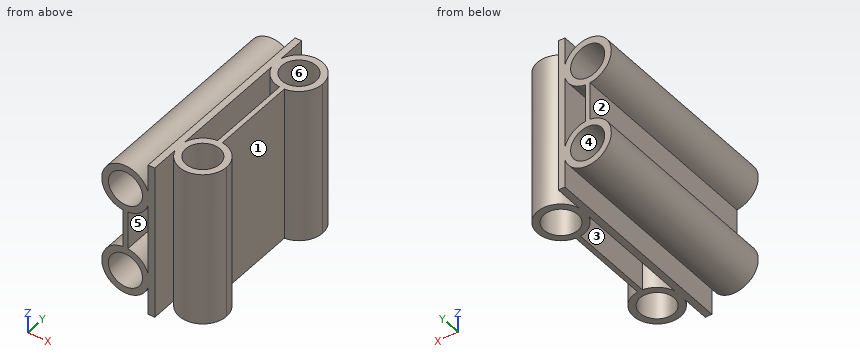
```python
from build123d import *

# Parameters (mm, degrees)
F2_W          = 7
F2_H          = 214
F3_DEPTH      = 82
F3_DEPTH_BACK = 82
F0_R          = 18
F4_DEPTH      = 107
F4_DEPTH_BACK = 107
F1_R          = 18
F5_DEPTH      = 82
F5_DEPTH_BACK = 82


with BuildPart() as f3:
    # F2 (on Top) → F3 (new body, two sides)
    with BuildSketch(Plane.XY) as f3_sk:
        with Locations((-27.5, 0)):
            Rectangle(F2_W, F2_H)
    extrude(amount=F3_DEPTH)
    extrude(f3_sk.sketch, amount=-F3_DEPTH_BACK)

    # F0 (on Front) → F4 (join, two sides)
    with BuildSketch(Plane.XZ) as f4_sk:
        with BuildLine():
            ThreePointArc((-52.5, 20.125314), (-36.459504, 28.22949), (-30, 45))
            ThreePointArc((-30, 45), (-71.77051, 63.540496), (-57.5, 20.125314))
            Line((-57.5, 20.125314), (-52.5, 20.125314))
        make_face()
        with Locations((-55, 45)):
            Circle(F0_R, mode=Mode.SUBTRACT)
        with BuildLine():
            Line((-52.5, -20.125314), (-57.5, -20.125314))
            ThreePointArc((-57.5, -20.125314), (-71.77051, -63.540496), (-30, -45))
            ThreePointArc((-30, -45), (-36.459504, -28.22949), (-52.5, -20.125314))
        make_face()
        with Locations((-55, -45)):
            Circle(F0_R, mode=Mode.SUBTRACT)
        with BuildLine():
            Line((-52.5, 20.125314), (-57.5, 20.125314))
            ThreePointArc((-57.5, 20.125314), (-55, 20), (-52.5, 20.125314))
        make_face()
        with BuildLine():
            ThreePointArc((-52.5, 20.125314), (-55, 20), (-57.5, 20.125314))
            Line((-57.5, 20.125314), (-57.5, -20.125314))
            ThreePointArc((-57.5, -20.125314), (-55, -20), (-52.5, -20.125314))
            Line((-52.5, -20.125314), (-52.5, 20.125314))
        make_face()
        with BuildLine():
            ThreePointArc((-52.5, -20.125314), (-55, -20), (-57.5, -20.125314))
            Line((-57.5, -20.125314), (-52.5, -20.125314))
        make_face()
    extrude(amount=F4_DEPTH)
    extrude(f4_sk.sketch, amount=-F4_DEPTH_BACK)

    # F1 (on Top) → F5 (join, two sides)
    with BuildSketch(Plane.XY) as f5_sk:
        with BuildLine():
            ThreePointArc((2.5, 45.125314), (18.540496, 53.22949), (25, 70))
            ThreePointArc((25, 70), (-16.77051, 88.540496), (-2.5, 45.125314))
            Line((-2.5, 45.125314), (2.5, 45.125314))
        make_face()
        with Locations((0, 70)):
            Circle(F1_R, mode=Mode.SUBTRACT)
        with BuildLine():
            ThreePointArc((2.5, 45.125314), (0, 45), (-2.5, 45.125314))
            Line((-2.5, 45.125314), (-2.5, -45.125314))
            ThreePointArc((-2.5, -45.125314), (0, -45), (2.5, -45.125314))
            Line((2.5, -45.125314), (2.5, 45.125314))
        make_face()
        with BuildLine():
            Line((2.5, 45.125314), (-2.5, 45.125314))
            ThreePointArc((-2.5, 45.125314), (0, 45), (2.5, 45.125314))
        make_face()
        with BuildLine():
            Line((2.5, -45.125314), (-2.5, -45.125314))
            ThreePointArc((-2.5, -45.125314), (-16.77051, -88.540496), (25, -70))
            ThreePointArc((25, -70), (18.540496, -53.22949), (2.5, -45.125314))
        make_face()
        with Locations((0, -70)):
            Circle(F1_R, mode=Mode.SUBTRACT)
        with BuildLine():
            ThreePointArc((2.5, -45.125314), (0, -45), (-2.5, -45.125314))
            Line((-2.5, -45.125314), (2.5, -45.125314))
        make_face()
    extrude(amount=F5_DEPTH)
    extrude(f5_sk.sketch, amount=-F5_DEPTH_BACK)


solid = f3.part
```
For this review, take the finished solid that the model builds, in its own axes (mm). Face numbers are marked on the shaded views. A direction names the side the tool comes from. Round coordinates to 2 decimals unless told otherwise and drop trailing zeros. Write each loop counter-clockwise with the first axis right and the second up, starting at its lowest first coordinate (ties: lowest second). Pieces come first, ordered by that corner, then holes. Notation, with made-up numbers: M 0,-16 L 13,-16 A21 cw 13,17 Z; hole C 30.5,52.5 d8. An arc over 180 degrees is marked long. One line per item, written item: value. Start each with the question number.
(1) We need section C-C (y = 24.5). Give the boundary of the cut face in (x, z), and give its area (3 significant figures).
(2) The part is to be moulded in two halves that separate along Y. For the marked faces 5 and 6, say which applies: released by +Y, released by -Y, zero draft, split by the parting line, or undercut.
(3) Insertion check: pin 1 (4 mm diameter, centred on y = -16, z = 56.5, fed in from +X); pin 2 (3 mm diameter, centred on x = -13.5, z = 30.5, fed in from -Y); pin 3 (10 mm diameter, centred on y = -54, z = 55, fed in from -X). Each pin has a flat end and moves straight along its axis. Give the tip position at first contact, or say it passes through.
(4) Machinability: for the marked faces 1, 2, 3 and 4, which of the approach directions +Z, -Z, +X, -X, +Y, -Y give a long, thin tool a straight path to every point of the face, cutting with its end or side? Answer none if there is none.
(5) We need section A-A (z = -8). Give the boundary of the cut face in (x, y).
(6) Wall thickness on line 1 (Z direction, x = -55, y = -40.5); line 2 (X direction, y = -27.5, z = -10); line 3 (Y direction, x = 0, z = 2): over which ranges is each line inside the solid? List them lowest first.
(7) We need section D-D (y = -85). Give the boundary of the cut face in (x, z), and give its area (3 significant figures).
(8) We need section B-B (x = -55). Give the boundary of the cut face in (y, z), and give its area (3 significant figures).
Result:
1. outline: M -57.5,-20.13 A25 ccw long -31,-52 L -31,-82 L -24,-82 L -24,82 L -31,82 L -31,52 A25 ccw long -57.5,20.13 Z; M -2.5,-82 L 2.5,-82 L 2.5,82 L -2.5,82 Z; hole C -55,-45 d36; hole C -55,45 d36; hole M -52.5,-20.13 A25 cw -31,-38 L -31,38 A25 cw -52.5,20.13 Z
1. area: 4,040 mm²
2. face 5: zero draft
2. face 6: undercut
3. pin 1: x = 2.5
3. pin 2: y = -91.93
3. pin 3: x = -79.49
4. face 1: +Z, -Z, +X
4. face 2: -X, +Y, -Y
4. face 3: +Z, -Z
4. face 4: +Y, -Y
5. outline: M -57.5,-107 L -52.5,-107 L -52.5,107 L -57.5,107 Z; M -31,-107 L -24,-107 L -24,-77 A25 ccw long 2.5,-45.13 L 2.5,45.13 A25 ccw long -24,77 L -24,107 L -31,107 Z; hole M -24,-63 A25 cw -2.5,-45.13 L -2.5,45.13 A25 cw -24,63 Z; hole C 0,-70 d36; hole C 0,70 d36
6. line 1: -70 to -63, -27 to 27, 63 to 70
6. line 2: -57.5 to -52.5, -31 to -24, -2.5 to 2.5
6. line 3: -95 to -88, -52 to 52, 88 to 95
7. outline: M -57.5,-20.13 A25 ccw long -31,-52 L -31,-82 L -24,-82 L -24,82 L -31,82 L -31,52 A25 ccw long -57.5,20.13 Z; M -20,-82 L -9.95,-82 L -9.95,82 L -20,82 Z; M 9.95,-82 L 20,-82 L 20,82 L 9.95,82 Z; hole C -55,-45 d36; hole C -55,45 d36; hole M -52.5,-20.13 A25 cw -31,-38 L -31,38 A25 cw -52.5,20.13 Z
7. area: 6,520 mm²
8. outline: M -107,-70 L 107,-70 L 107,-63 L -107,-63 Z; M -107,-27 L 107,-27 L 107,27 L -107,27 Z; M -107,63 L 107,63 L 107,70 L -107,70 Z
8. area: 14,600 mm²
